Could you check a few things on this model? Use its own coordinates, in mm. A direction names the side the tool comes from. Coordinates: 2 decimals unless noted, no trailing zeros. Order: outer loops, then holes, each group sorted by start corner. A loop starts at its lowest first (then second) coordinate and runs counter-clockwise, first axis right, second up. Notation, with made-up numbers: (-39.75, 36) - (-20.75, 36) arc R18 ccw to (-20.75, 40) - close; hole circle Ø11 at (50.25, 9.25). An arc over 180 degrees is marked (long way). One line per item, written item: value.
Autodesk Inventor part; units mm, degrees
ref_plane "YZ Plane" through (0, 0, 0) normal (1, 0, 0) x (0, 1, 0)
ref_plane "XZ Plane" through (0, 0, 0) normal (0, 1, 0) x (-1, 0, 0)
ref_plane "XY Plane" through (0, 0, 0) normal (0, 0, 1) x (1, 0, 0)
sketch "Sketch1" plane through (0, 0, 0) normal (0, 0, 1) x (1, 0, 0)
  line L0 (0, 0) -> (-100, 0)
  line L1 (-100, 0) -> (-100, 50)
  line L2 (-100, 50) -> (0, 50)
  line L3 (0, 50) -> (0, 0)
  line L4 (-93.25, 46.75) -> (-76.75, 46.75)
  line L5 (-75, 45) -> (-75, 45)
  line L6 (-76.75, 43.25) -> (-93.25, 43.25)
  line L7 (-95, 45) -> (-95, 45)
  line L8 (-93.25, 6.75) -> (-76.75, 6.75)
  line L9 (-75, 5) -> (-75, 5)
  line L10 (-76.75, 3.25) -> (-93.25, 3.25)
  line L11 (-95, 5) -> (-95, 5)
  arc A0 (-93.25, 46.75) -> (-95, 45) centre (-93.25, 45) ccw
  arc A1 (-95, 45) -> (-93.25, 43.25) centre (-93.25, 45) ccw
  arc A2 (-75, 45) -> (-76.75, 46.75) centre (-76.75, 45) ccw
  arc A3 (-76.75, 43.25) -> (-75, 45) centre (-76.75, 45) ccw
  arc A4 (-75, 5) -> (-76.75, 6.75) centre (-76.75, 5) ccw
  arc A5 (-93.25, 6.75) -> (-95, 5) centre (-93.25, 5) ccw
  arc A6 (-95, 5) -> (-93.25, 3.25) centre (-93.25, 5) ccw
  arc A7 (-76.75, 3.25) -> (-75, 5) centre (-76.75, 5) ccw
  line L12 (0, 55) -> (-15, 55)
  line L13 (-15, 55) -> (-15, -5)
  line L14 (-15, -5) -> (0, -5)
  line L15 (0, -5) -> (0, 55)
  line L16 (-70, 50) -> (-15, 50)
  line L17 (-15, 50) -> (-15, 35)
  line L18 (-15, 35) -> (-70, 35)
  line L19 (-70, 35) -> (-70, 50)
  line L20 (-70, 0) -> (-15, 0)
  line L21 (-15, 0) -> (-15, 15)
  line L22 (-15, 15) -> (-70, 15)
  line L23 (-70, 15) -> (-70, 0)
  point P0 (-75, 43.25)
  point P1 (-75, 46.75)
  point P2 (-95, 43.25)
  point P3 (-95, 6.75)
  point P4 (-75, 3.25)
  point P5 (-75, 6.75)
  dimension "d0" = 100
  dimension "d1" = 50
  dimension "d2" = 20
  dimension "d3" = 3.5
  dimension "d4" = 3.5
  dimension "d5" = 36.5
  dimension "d6" = 3.25
  dimension "d7" = 5
  dimension "d8" = 1.75
  dimension "d11" = 15
  dimension "d12" = 60
  dimension "d13" = 15
  dimension "d14" = 15
  dimension "d17" = 55
  dimension "d18" = 15
  dimension "d19" = 5
extrude "Extrusion1" add sketch "Sketch1" along normal blind 2 contours L15 L14 L13 L0 | L0 L13 L2 L3 | L2 L13 L12 L15 | L0 L1 L2 L19 L18 L13 L22 L23
fillet "Fillet1" radius 4 12 edges at (-70, 50, 1) (-70, 35, 1) (-100, 50, 1) (-100, 0, 1) (-70, 0, 1) (-70, 15, 1) (-15, 15, 1) (-15, 35, 1) (-15, 55, 1) (0, 55, 1) (0, -5, 1) (-15, -5, 1)
sketch "Sketch2" plane through (0, 0, 2) normal (0, 0, 1) x (1, 0, 0)
  line L0 (-7.5, 49) -> (-7.5, 49)
  line L1 (-4.4, 45.9) -> (-4.4, 42.1)
  line L2 (-7.5, 39) -> (-7.5, 39)
  line L3 (-10.6, 42.1) -> (-10.6, 45.9)
  line L4 (-7.5, 11) -> (-7.5, 11)
  line L5 (-4.4, 7.9) -> (-4.4, 4.1)
  line L6 (-7.5, 1) -> (-7.5, 1)
  line L7 (-10.6, 4.1) -> (-10.6, 7.9)
  line L8 (0, -1) -> (0, 51)
  line L9 (-4, 55) -> (-11, 55)
  line L10 (-11, -5) -> (-4, -5)
  arc A0 (-7.5, 49) -> (-10.6, 45.9) centre (-7.5, 45.9) ccw
  arc A1 (-4.4, 45.9) -> (-7.5, 49) centre (-7.5, 45.9) ccw
  arc A2 (-7.5, 39) -> (-4.4, 42.1) centre (-7.5, 42.1) ccw
  arc A3 (-10.6, 42.1) -> (-7.5, 39) centre (-7.5, 42.1) ccw
  arc A4 (-7.5, 11) -> (-10.6, 7.9) centre (-7.5, 7.9) ccw
  arc A5 (-7.5, 1) -> (-4.4, 4.1) centre (-7.5, 4.1) ccw
  arc A6 (-4.4, 7.9) -> (-7.5, 11) centre (-7.5, 7.9) ccw
  arc A7 (-10.6, 4.1) -> (-7.5, 1) centre (-7.5, 4.1) ccw
  point P0 (0, 0)
  point P1 (-4.4, 39)
  point P2 (-4.4, 49)
  point P3 (-10.6, 39)
  point P4 (-4.4, 1)
  point P5 (-4.4, 11)
  point P6 (-10.6, 1)
  point P7 (-7.5, 49)
  point P8 (-7.5, 1)
  point P9 (-7.5, 1)
  dimension "d21" = 6.2
  dimension "d22" = 10
  dimension "d23" = 6.2
  dimension "d24" = 10
  dimension "d25" = 4.4
  dimension "d26" = 4.4
  dimension "d27" = 6
  dimension "d28" = 6
  dimension "d29" = 3.1
extrude "Extrusion2" cut sketch "Sketch2" against normal blind 2
sketch "Sketch3" plane through (0, 0, 2) normal (0, 0, 1) x (1, 0, 0)
  line L0 (0, -1) -> (0, 51)
  line L1 (-100, 24) -> (-100, 26)
  line L2 (0, 26) -> (0, 24)
  line L3 (-11, 55) -> (-4, 55)
  line L4 (0, 51) -> (0, 39)
  line L5 (-15, 39) -> (-15, 51)
  line L6 (-4, -5) -> (-11, -5)
  line L7 (-15, -1) -> (-15, 11)
  line L8 (0, 11) -> (0, -1)
  line L9 (-96, 50) -> (-74, 50)
  line L10 (-70, 46) -> (-70, 39)
  line L11 (-100, 39) -> (-100, 46)
  line L12 (-100, 46) -> (-100, 4)
  line L13 (-74, 0) -> (-96, 0)
  line L14 (-100, 4) -> (-100, 11)
  line L15 (-70, 11) -> (-70, 4)
  arc A0 (-96, 50) -> (-100, 46) centre (-96, 46) ccw
  arc A1 (-70, 46) -> (-74, 50) centre (-74, 46) ccw
  arc A2 (-100, 39) -> (-96, 35) centre (-96, 39) ccw
  arc A3 (-74, 35) -> (-70, 39) centre (-74, 39) ccw
  arc A4 (-96, 15) -> (-100, 11) centre (-96, 11) ccw
  arc A5 (-100, 4) -> (-96, 0) centre (-96, 4) ccw
  arc A6 (-74, 0) -> (-70, 4) centre (-74, 4) ccw
  arc A7 (-70, 11) -> (-74, 15) centre (-74, 11) ccw
  arc A8 (-11, 15) -> (-15, 11) centre (-11, 11) ccw
  arc A9 (0, 11) -> (-4, 15) centre (-4, 11) ccw
  arc A10 (-4, -5) -> (0, -1) centre (-4, -1) ccw
  arc A11 (-15, -1) -> (-11, -5) centre (-11, -1) ccw
  arc A12 (-15, 39) -> (-11, 35) centre (-11, 39) ccw
  arc A13 (-4, 35) -> (0, 39) centre (-4, 39) ccw
  arc A14 (0, 51) -> (-4, 55) centre (-4, 51) ccw
  arc A15 (-11, 55) -> (-15, 51) centre (-11, 51) ccw
  line L16 (-100, 26) -> (-86, 26)
  line L17 (-86, 35) -> (-86, 26)
  line L18 (-86, 24) -> (-86, 15)
  line L19 (-86, 24) -> (-100, 24)
  line L20 (-84, 15) -> (-84, 24)
  line L21 (-84, 26) -> (-84, 35)
  line L22 (-96, 15) -> (-86, 15)
  line L23 (-84, 15) -> (-74, 15)
  line L24 (-74, 35) -> (-84, 35)
  line L25 (-86, 35) -> (-96, 35)
  line L26 (-4, 35) -> (-6.5, 35)
  line L27 (-8.5, 35) -> (-11, 35)
  line L28 (-84, 26) -> (-8.5, 26)
  line L29 (-6.5, 26) -> (0, 26)
  line L30 (-8.5, 35) -> (-8.5, 26)
  line L31 (-8.5, 24) -> (-8.5, 15)
  line L32 (-6.5, 15) -> (-6.5, 24)
  line L33 (-6.5, 26) -> (-6.5, 35)
  line L34 (0, 24) -> (-6.5, 24)
  line L35 (-8.5, 24) -> (-84, 24)
  line L36 (-11, 15) -> (-8.5, 15)
  line L37 (-6.5, 15) -> (-4, 15)
  line L38 (-10.6, 45.9) -> (-10.6, 42.1)
  line L39 (-10.6, 45.9) -> (-10.6, 42.1)
  arc A16 (-10.6, 42.1) -> (-4.4, 42.1) centre (-7.5, 42.1) ccw
  arc A17 (-10.6, 42.1) -> (-4.4, 42.1) centre (-7.5, 42.1) ccw
  arc A18 (-4.4, 45.9) -> (-10.6, 45.9) centre (-7.5, 45.9) ccw
  arc A19 (-4.4, 45.9) -> (-10.6, 45.9) centre (-7.5, 45.9) ccw
  line L40 (-4.4, 45.9) -> (-4.4, 42.1)
  arc A20 (-4.4, 7.9) -> (-10.6, 7.9) centre (-7.5, 7.9) ccw
  arc A21 (-4.4, 7.9) -> (-10.6, 7.9) centre (-7.5, 7.9) ccw
  arc A22 (-10.6, 4.1) -> (-4.4, 4.1) centre (-7.5, 4.1) ccw
  arc A23 (-10.6, 4.1) -> (-4.4, 4.1) centre (-7.5, 4.1) ccw
  line L41 (-10.6, 7.9) -> (-10.6, 4.1)
  line L42 (-10.6, 7.9) -> (-10.6, 4.1)
  line L43 (-4.4, 4.1) -> (-4.4, 7.9)
  line L44 (-4.4, 4.1) -> (-4.4, 7.9)
  arc A24 (-93.25, 46.75) -> (-93.25, 43.25) centre (-93.25, 45) ccw
  line L45 (-93.25, 46.75) -> (-76.75, 46.75)
  line L46 (-93.25, 46.75) -> (-76.75, 46.75)
  arc A25 (-93.25, 46.75) -> (-93.25, 43.25) centre (-93.25, 45) ccw
  arc A26 (-76.75, 43.25) -> (-76.75, 46.75) centre (-76.75, 45) ccw
  line L47 (-76.75, 43.25) -> (-93.25, 43.25)
  line L48 (-93.25, 43.25) -> (-76.75, 43.25)
  arc A27 (-93.25, 6.75) -> (-93.25, 3.25) centre (-93.25, 5) ccw
  line L49 (-93.25, 6.75) -> (-76.75, 6.75)
  arc A28 (-76.75, 3.25) -> (-76.75, 6.75) centre (-76.75, 5) ccw
  arc A29 (-76.75, 3.25) -> (-76.75, 6.75) centre (-76.75, 5) ccw
  line L50 (-76.75, 3.25) -> (-93.25, 3.25)
  point P0 (0, 0)
  point P1 (0, 25)
  point P2 (0, 35)
  point P3 (0, 55)
  point P4 (0, -5)
  point P5 (-15, 15)
  point P6 (-15, -5)
  point P7 (-70, 35)
  point P8 (-100, 35)
  point P9 (-70, 0)
  point P10 (-100, 15)
  point P11 (-85, 35)
  point P12 (-7.5, 35)
  dimension "d32" = 100
  dimension "d33" = 2
  dimension "d35" = 20
  dimension "d36" = 20
  dimension "d37" = 4
extrude "Extrusion3" add sketch "Sketch3" along normal blind 4 contours A10 L6 A11 L7 A8 L36 L31 L35 L20 L23 A7 L15 A6 L13 A5 L12 A4 L22 L18 L19 L1 L16 L17 L25 A2 L11 A0 L9 A1 L10 A3 L24 L21 L28 L30 L27 A12 L5 A15 L3 A14 L0 A13 L26 L33 L29 L34 L32 L37 A9
sketch "Sketch5" plane through (0, 0, 6) normal (0, 0, 1) x (1, 0, 0)
  line L0 (-93.25, 6.75) -> (-76.75, 6.75)
  arc A0 (-76.75, 3.25) -> (-76.75, 6.75) centre (-76.75, 5) ccw
  arc A1 (-93.25, 6.75) -> (-93.25, 3.25) centre (-93.25, 5) ccw
  line L1 (-76.75, 3.25) -> (-93.25, 3.25)
  arc A2 (-76.75, 2) -> (-76.75, 8) centre (-76.75, 5) ccw
  arc A3 (-93.25, 8) -> (-93.25, 2) centre (-93.25, 5) ccw
  line L2 (-76.75, 2) -> (-93.25, 2)
  line L3 (-93.25, 8) -> (-76.75, 8)
  line L4 (-70, 0) -> (-70, 7.5)
  line L5 (-70, 4) -> (-70, 11)
  arc A4 (-76.75, 42) -> (-76.75, 48) centre (-76.75, 45) ccw
  arc A5 (-93.25, 48) -> (-93.25, 42) centre (-93.25, 45) ccw
  line L6 (-76.75, 42) -> (-93.25, 42)
  line L7 (-93.25, 48) -> (-76.75, 48)
  point P0 (-75, 5)
  point P1 (-75, 45)
  dimension "d68" = 6
  dimension "d69" = 6
  dimension "d72" = 40
extrude "Extrusion4" cut sketch "Sketch5" against normal blind 3.2 contours L0 A0 L1 A1 | L2 A3 L3 A2 | L6 A5 L7 A4
equation "\"d26\" = d25"
properties part number "panel_holder"
Item 1: I want a section at B-B on y = 18. Please give me the cut outline in (x, z).
Conclusion:
outline: (-100, 0) - (0, 0) - (0, 2) - (-6.5, 2) - (-6.5, 6) - (-8.5, 6) - (-8.5, 2) - (-84, 2) - (-84, 6) - (-86, 6) - (-86, 2) - (-100, 2) - close
Item 2: I want a section at D-D on z = 4.4. Give the number of separate pieces and of enclosed holes in the cut face, then the cut area to 3 significant figures.
Conclusion:
separate pieces: 1
enclosed holes: 4
area: 1,360 mm²
Item 3: I'm going to push flat-ended pins straight in: pin 1 Ø1.6 at (x, z) = (-42, 0.5) entering from +Y; pin 2 Ø2 at (y, z) = (21, 5) entering from +X; pin 3 Ø1.5 at (x, z) = (-17, 2) entering from +Y; pin 4 Ø1 at (y, z) = (27, 0.5) entering from +X. Where does each tip first touch, or does it pass through?
Conclusion:
pin 1: y = 35
pin 2: x = -6.5
pin 3: y = 36.1
pin 4: x = 0
Item 4: For faces 1 (the face through (-85, 43.25, 1)), 2 (the face through (-3, 26, 4)), 3 (the face through (-84, 19, 4)), 4 (the face through (-16.141, 13.797, 1.014)), which set-ups out of +Z, -Z, +X, -X, +Y, -Y let a thin tool reach every point of the face, with its end or its side?
Conclusion:
face 1: +Z, -Z
face 2: +Z, +X
face 3: +Z
face 4: +Z, -Z, -Y
Item 5: I want a section at C-C on y = 38. Please give me the cut outline in (x, z).
Conclusion:
outline: (-100, 0) - (-69.87, 0) - (-69.87, 2) - (-70.13, 2) - (-70.13, 6) - (-99.87, 6) - (-99.87, 2) - (-100, 2) - close; (-15.13, 0) - (0, 0) - (0, 2) - (-0.13, 2) - (-0.13, 6) - (-14.87, 6) - (-14.87, 2) - (-15.13, 2) - close
Item 6: If I drill on probe 1 along Y at (x, z) = (-91, 4.75); probe 2 along Y at (x, z) = (-13, 4.8); probe 3 along X at (y, z) = (43.5, 4.1), over which ranges is the centre line in solid material (lowest first)?
Conclusion:
probe 1: 0 to 2, 8 to 15, 24 to 26, 35 to 42, 48 to 50
probe 2: -4.46 to 14.46, 24 to 26, 35.54 to 54.46
probe 3: -100 to -95.85, -74.15 to -70, -15 to -10.6, -4.4 to 0
Item 7: I want a section at A-A on x = -62.5. Please give me the cut outline in (y, z), then the cut area to 3 significant figures.
Conclusion:
outline: (15, 0) - (35, 0) - (35, 2) - (26, 2) - (26, 6) - (24, 6) - (24, 2) - (15, 2) - close
area: 48.0 mm²
Item 8: Thinking about a two-plate mould opening in X: for faces 5 (the face through (-91, 15, 4)), 6 (the face through (-86, 20, 4)), 7 (the face through (-10, 15, 4)), 8 (the face through (-71.141, 1.203, 2.958)), which applies, pulls with the +X half, pulls with the -X half, needs draft (parallel to the pull), parting line crosses it, or undercut?
Conclusion:
face 5: needs draft
face 6: pulls with the -X half
face 7: undercut
face 8: undercut
